```python
from build123d import *

# Parameters (mm, degrees)
F1_DEPTH = 22.225
F2_R     = 6.35
F3_R     = 15.875
F4_R     = 11.90625
F5_DEPTH = 25.4


with BuildPart() as f1:
    # F0 (on Front) → F1 (new body, symmetric)
    with BuildSketch(Plane.XZ):
        Polygon((-41.275, 41.275), (41.275, 41.275), (41.275, -12.7), (50.8, -12.7), (50.8, 50.8), (41.275, 50.8), (-41.275, 50.8), (-50.8, 50.8), (-50.8, -12.7), (-41.275, -12.7), align=None)
    extrude(amount=F1_DEPTH, both=True)

    # F2
    f2_edges = [f1.edges().sort_by_distance(p)[0] for p in [
        (-41.275, 0, 41.275),
        (41.275, 0, 41.275),
    ]]
    fillet(f2_edges, radius=F2_R)

    # F3
    f3_edges = [f1.edges().sort_by_distance(p)[0] for p in [
        (50.8, 0, 50.8),
        (-50.8, 0, 50.8),
    ]]
    fillet(f3_edges, radius=F3_R)

    # F4 (on face) → F5 (cut)
    with BuildSketch(Plane.XY.offset(50.8)):
        Circle(F4_R)
    extrude(amount=-F5_DEPTH, mode=Mode.SUBTRACT)


solid = f1.part
```
Source: CAD feature listing. Evaluate the final solid. Frame: model axes, mm. A direction names the side the tool comes from. Round coordinates to 2 decimals unless told otherwise and drop trailing zeros. Loops run counter-clockwise (first coordinate to the right, second up) from the corner with the lowest first, then second, coordinate; pieces in that order, holes last. Notation, with made-up numbers: M 14,-23 L 27,-23 A27 ccw 27,5 Z; hole C 82.5,74 d4. An arc over 180 degrees is marked long. Use a Markdown table: item, result. Add a question column.
1. Line query: line 1 (Y direction, x = 0, z = 47) (3 decimals); line 2 (X direction, y = -2, z = 34) (3 decimals); line 3 (Z direction, x = 10, y = -8) (3 decimals). Output: solid intervals per line, ascending.
2. Mould query, pull axis X, two halves, no side actions, for faces 3 (the flat face through (-50.8, 0, 11)), 4 (the flat face through (50.8, 0, 11)), 5 (the flat face through (46, 0, -12.7)), 6 (the cylindrical face through (-39.37, 0.31, 39.46)). Classes: pulls with the +X half, pulls with the -X half, needs draft (parallel to the pull), parting line crosses it, or undercut.
3. Reachability of faces 1 (the flat face through (8, -10, 50.8)), 2 (the flat face through (7, -10, 41.275)) from +Z, -Z, +X, -X, +Y, -Y: full face, straight path, thin tool, end or side. Return the list, or none.
4. Section query C-C on x = 0. Return the cut outline in (y, z) (3 decimals).
5. Section query D-D on y = -17. Return the cut outline in (x, z) (3 decimals), then the cut area to 3 significant figures.
6. Section query B-B on z = 29. Return the cut outline in (x, y) (3 decimals), then the cut area to 3 significant figures.
7. Section query A-A on y = 0. Return the cut outline in (x, z) (3 decimals), then the cut area to 3 significant figures.
8. Contact query for flat-ended pins moving along their axis: P1, Ø14.5, axis at x = 0, y = 0, coming from the -Z side; P2, Ø22, axis at x = 3.5, y = -8, coming from the -Z side (3 decimals); P3, Ø5, axis at x = -35, y = -4, coming from the -Z side; P4, Ø10, axis at x = 2.5, z = 37.5, coming from the -Y side (3 decimals). Output: stop coordinate, or through.
Reported:
| question | item | result |
|---|---|---|
| 1 | line 1 | y = -22.225 to -11.906, 11.906 to 22.225 |
| 1 | line 2 | x = -50.8 to -41.275, 41.275 to 50.8 |
| 1 | line 3 | z = 41.275 to 50.8 |
| 2 | face 3 | pulls with the -X half |
| 2 | face 4 | pulls with the +X half |
| 2 | face 5 | needs draft |
| 2 | face 6 | undercut |
| 3 | face 1 | +Z, +X, -X, +Y, -Y |
| 3 | face 2 | -Z, +Y, -Y |
| 4 | outline | M -22.225,41.275 L -11.906,41.275 L -11.906,50.8 L -22.225,50.8 Z; M 11.906,41.275 L 22.225,41.275 L 22.225,50.8 L 11.906,50.8 Z |
| 5 | outline | M -50.8,-12.7 L -41.275,-12.7 L -41.275,34.925 A6.35 cw -34.925,41.275 L 34.925,41.275 A6.35 cw 41.275,34.925 L 41.275,-12.7 L 50.8,-12.7 L 50.8,34.925 A15.875 ccw 34.925,50.8 L -34.925,50.8 A15.875 ccw -50.8,34.925 Z |
| 5 | area | 1,910 mm² |
| 6 | outline | M -50.8,-22.225 L -41.275,-22.225 L -41.275,22.225 L -50.8,22.225 Z; M 41.275,-22.225 L 50.8,-22.225 L 50.8,22.225 L 41.275,22.225 Z |
| 6 | area | 847 mm² |
| 7 | outline | M -50.8,-12.7 L -41.275,-12.7 L -41.275,34.925 A6.35 cw -34.925,41.275 L -11.906,41.275 L -11.906,50.8 L -34.925,50.8 A15.875 ccw -50.8,34.925 Z; M 11.906,41.275 L 34.925,41.275 A6.35 cw 41.275,34.925 L 41.275,-12.7 L 50.8,-12.7 L 50.8,34.925 A15.875 ccw 34.925,50.8 L 11.906,50.8 Z |
| 7 | area | 1,680 mm² |
| 8 | P1 | passes through |
| 8 | P2 | stops at z = 41.275 |
| 8 | P3 | stops at z = 40.73 |
| 8 | P4 | stops at y = -22.225 |
